Can you work these out from the model? Positions are in its coordinate system, mm. Face numbers are marked on the shaded views. A direction names the side the tool comes from. Give positions to 0.01 mm unless a question says otherwise; leave off trailing zeros. Order: outer loops, then holes, each group sorted by start corner. A loop starts at its lowest first (then second) coordinate and runs counter-clockwise, first axis right, second up. Notation, with made-up numbers: M 83.25,7 L 94.25,7 A19 cw 94.25,37 Z; hole C 30,14 d8. An arc over 180 degrees is marked long. Use one line per item in the form item = value. Start each with the question number.
1. I need wall thicknesses on L1, parallel to Y at x = 20.5, z = 11.5; L2, parallel to Y at x = 16.5, z = 5.5; L3, parallel to X at y = -15.5, z = 2. Which ranges of each line are inside material? Lowest first, please.
2. Will these pins go through, and if not, where does the flat tip stop? P1, Ø2, axis at y = 24, z = 9.5, coming from the -X side; P2, Ø2, axis at x = 20.5, y = -18, coming from the +Z side; P3, Ø4, axis at x = 20, y = 8, coming from the +Z side.
3. I want a section at B-B, the plane x = 20.5. List the corners of the cut face in (y, z) for me.
4. For the marked faces 1 and 2, which set-ups out of +Z, -Z, +X, -X, +Y, -Y let a thin tool reach every point of the face, with its end or its side?
5. I want a section at D-D, the plane z = 7. Count the separate pieces of the cut face and the enclosed holes in it, and give its area (3 significant figures).
6. I want a section at C-C, the plane y = 21. List the corners of the cut face in (x, z) for me, and give its area (3 significant figures).
7. We'd pull the mould along X, two halves only. Please class the marked faces 3, 4, 5 and 6: +X half, -X half, draft (parallel to the pull), parting line (faces both ways), or undercut.
8. I want a section at A-A, the plane y = -18. List the corners of the cut face in (x, z) for me.
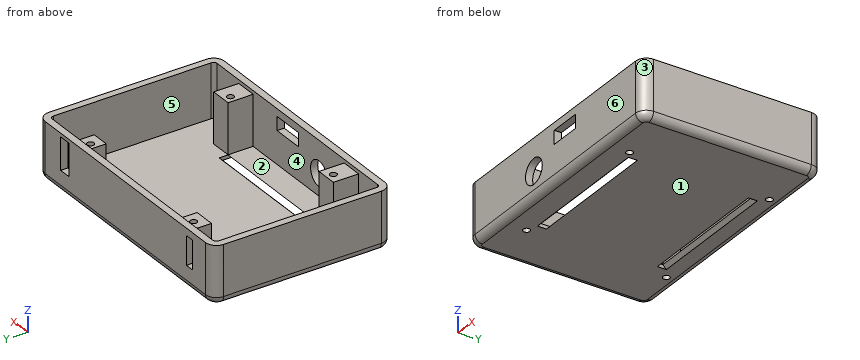
```python
from build123d import *

# Parameters (mm, degrees)
SKETCH1_W           = 73
SKETCH1_H           = 50
BOSS_EXTRUDE1_DEPTH = 1
SKETCH2_W           = 73
SKETCH2_H           = 50
SKETCH2_W_2         = 69
SKETCH2_H_2         = 46
BOSS_EXTRUDE2_DEPTH = 15
FILLET1_R           = 3
FILLET2_R           = 1
SKETCH3_W           = 9
SKETCH3_H           = 3.8
CUT_EXTRUDE1_DEPTH  = 2
SKETCH5_R           = 3.5
CUT_EXTRUDE2_DEPTH  = 2
SKETCH6_W           = 6
SKETCH6_H           = 5
SKETCH6_W_2         = 5
BOSS_EXTRUDE3_DEPTH = 14
SKETCH7_W           = 6
SKETCH7_H           = 7
BOSS_EXTRUDE4_DEPTH = 14
FILLET3_R           = 2
SKETCH8_W           = 2.5
SKETCH8_H           = 7.999199493
SKETCH8_W_2         = 3.5
SKETCH8_H_2         = 9
CUT_EXTRUDE3_DEPTH  = 63.387899545
SKETCH9_R           = 0.95
CUT_EXTRUDE4_DEPTH  = 47.714558812
SKETCH10_W          = 38
SKETCH10_H          = 1.5
CUT_EXTRUDE5_DEPTH  = 47.714558812
CHAMFER1_SIZE       = 1
CHAMFER2_SIZE       = 1


with BuildPart() as part:
    # Sketch1 → Boss-Extrude1 (new body)
    with BuildSketch(Plane.XY):
        Rectangle(SKETCH1_W, SKETCH1_H)
    extrude(amount=BOSS_EXTRUDE1_DEPTH)

    # Sketch2 → Boss-Extrude2 (add)
    with BuildSketch(Plane.XY.offset(1)):
        Rectangle(SKETCH2_W, SKETCH2_H)
        Rectangle(SKETCH2_W_2, SKETCH2_H_2, mode=Mode.SUBTRACT)
    extrude(amount=BOSS_EXTRUDE2_DEPTH)

    # Fillet1
    fillet1_edges = [part.edges().sort_by_distance(p)[0] for p in [
        (36.5, -25, 8),
        (-36.5, -25, 8),
        (-36.5, 25, 8),
        (36.5, 25, 8),
    ]]
    fillet(fillet1_edges, radius=FILLET1_R)

    # Fillet2
    fillet2_edges = [part.edges().sort_by_distance(p)[0] for p in [
        (34.5, 23, 8.5),
        (-34.5, 23, 8.5),
        (-34.5, -23, 8.5),
        (34.5, -23, 8.5),
    ]]
    fillet(fillet2_edges, radius=FILLET2_R)

    # Sketch3 → Cut-Extrude1 (cut)
    with BuildSketch(Plane.XZ.offset(25)):
        with Locations((4, 12)):
            Rectangle(SKETCH3_W, SKETCH3_H)
    extrude(amount=-CUT_EXTRUDE1_DEPTH, mode=Mode.SUBTRACT)

    # Sketch5 → Cut-Extrude2 (cut)
    with BuildSketch(Plane(origin=(0, -23, 0), x_dir=(1, 0, 0), z_dir=(0, 1, 0))):
        with Locations(Location((-8.976447348, -7, 0), (0, 0, 270))):
            Circle(SKETCH5_R)
    extrude(amount=-CUT_EXTRUDE2_DEPTH, mode=Mode.SUBTRACT)

    # Sketch6 → Boss-Extrude3 (add)
    with BuildSketch(Plane.XY.offset(1)):
        with Locations((-22.5, 20.5)):
            Rectangle(SKETCH6_W, SKETCH6_H)
        with Locations((21, 20.5)):
            Rectangle(SKETCH6_W_2, SKETCH6_H)
    extrude(amount=BOSS_EXTRUDE3_DEPTH)

    # Sketch7 → Boss-Extrude4 (add)
    with BuildSketch(Plane.XY.offset(1)):
        with Locations((21.5, -19.5)):
            Rectangle(SKETCH7_W, SKETCH7_H)
        with Locations((-22.5, -19.5)):
            Rectangle(SKETCH7_W, SKETCH7_H)
    extrude(amount=BOSS_EXTRUDE4_DEPTH)

    # Fillet3
    fillet3_edges = [part.edges().sort_by_distance(p)[0] for p in [
        (-36.5, 0, 0),
        (36.5, 0, 0),
        (0, -25, 0),
        (0, 25, 0),
        (35.621320344, -24.121320344, 0),
        (35.621320344, 24.121320344, 0),
        (-35.621320344, -24.121320344, 0),
        (-35.621320344, 24.121320344, 0),
    ]]
    fillet(fillet3_edges, radius=FILLET3_R)

    # Sketch8 → Cut-Extrude3 (cut, through all)
    with BuildSketch(Plane.XZ.offset(-23)):
        with Locations((-26.75, 9.999599746)):
            Rectangle(SKETCH8_W, SKETCH8_H)
        with Locations((25.25, 10.5)):
            Rectangle(SKETCH8_W_2, SKETCH8_H_2)
    extrude(amount=-CUT_EXTRUDE3_DEPTH, mode=Mode.SUBTRACT)

    # Sketch9 → Cut-Extrude4 (cut, through all)
    with BuildSketch(Plane.XY.offset(15)):
        with Locations((-22.5, 21)):
            Circle(SKETCH9_R)
        with Locations((20.5, 21)):
            Circle(SKETCH9_R)
        with Locations((20.5, -18)):
            Circle(SKETCH9_R)
        with Locations((-22.5, -18)):
            Circle(SKETCH9_R)
    extrude(amount=-CUT_EXTRUDE4_DEPTH, mode=Mode.SUBTRACT)

    # Sketch10 → Cut-Extrude5 (cut, through all)
    with BuildSketch(Plane.XY.offset(1)):
        with Locations((-0.5, 17.25)):
            Rectangle(SKETCH10_W, SKETCH10_H)
        with Locations((-0.5, -15.25)):
            Rectangle(SKETCH10_W, SKETCH10_H)
    extrude(amount=-CUT_EXTRUDE5_DEPTH, mode=Mode.SUBTRACT)

    # Chamfer1
    chamfer1_edges = [part.edges().sort_by_distance(p)[0] for p in [
        (-0.5, -16, 0),
        (-0.5, 18, 0),
    ]]
    chamfer(chamfer1_edges, length=CHAMFER1_SIZE - 0.0001)  # a hair under: the kernel refuses the full size

    # Chamfer2
    chamfer2_edges = [part.edges().sort_by_distance(p)[0] for p in [
        (-0.5, 16.5, 1),
        (-0.5, -14.5, 1),
    ]]
    chamfer(chamfer2_edges, length=CHAMFER2_SIZE - 0.0001)  # a hair under: the kernel refuses the full size


solid = part.part
```
Check result:
q1.L1 = -25 to -18.95, -17.05 to -16, 18 to 20.05, 21.95 to 25
q1.L2 = -25 to -23, 23 to 25
q1.L3 = -36.5 to -34.5, 34.5 to 36.5
q2.P1 = -36.33
q2.P2 = 15
q2.P3 = 1
q3.outline = M -25,2 A2 ccw -23,0 L -18.95,0 L -18.95,15 L -23,15 L -23,16 L -25,16 Z; M -17.05,0 L 20.05,0 L 20.05,15 L 18,15 L 18,1 L -16,1 L -16,15 L -17.05,15 Z; M 21.95,0 L 23,0 A2 ccw 25,2 L 25,16 L 23,16 L 23,15 L 21.95,15 Z
q4.face_1 = -Z, +X, -X, +Y, -Y
q4.face_2 = +Z
q5.separate_pieces = 3
q5.enclosed_holes = 4
q5.area = 571 mm2
q6.outline = M -36.5,2 A2 ccw -34.5,0 L -23.45,0 L -23.45,15 L -25.5,15 L -25.5,1 L -34.5,1 L -34.5,16 L -36.5,16 Z; M -21.55,0 L 19.55,0 L 19.55,15 L 18.5,15 L 18.5,1 L -19.5,1 L -19.5,15 L -21.55,15 Z; M 21.45,0 L 34.5,0 A2 ccw 36.5,2 L 36.5,16 L 34.5,16 L 34.5,1 L 23.5,1 L 23.5,15 L 21.45,15 Z
q6.area = 228 mm2
q7.face_3 = +X half
q7.face_4 = undercut
q7.face_5 = undercut
q7.face_6 = draft
q8.outline = M -36.5,2 A2 ccw -34.5,0 L -23.45,0 L -23.45,15 L -25.5,15 L -25.5,1 L -34.5,1 L -34.5,16 L -36.5,16 Z; M -21.55,0 L 19.55,0 L 19.55,15 L 18.5,15 L 18.5,1 L -19.5,1 L -19.5,15 L -21.55,15 Z; M 21.45,0 L 34.5,0 A2 ccw 36.5,2 L 36.5,16 L 34.5,16 L 34.5,1 L 24.5,1 L 24.5,15 L 21.45,15 Z
